from build123d import *

# Parameters (mm, degrees)
SKETCH_1_R          = 2.1
EXTRUDE_1_DEPTH     = 3
FILLET_1_R          = 3
SKETCH_2_W          = 9
SKETCH_2_H          = 5
CUT_EXTRUDE_1_DEPTH = 3
SKETCH_3_R          = 1.5
CUT_EXTRUDE_2_DEPTH = 10
FILLET_2_R          = 1.5


with BuildPart() as part:
    # 草图1 → 凸台-拉伸1 (new body)
    with BuildSketch(Plane(origin=(0, 0, 0), x_dir=(1, 0, 0), z_dir=(0, 1, 0))):
        Polygon((33, 10), (-33, 10), (-33, -10), (-10, -60), (10, -60), (33, -10), align=None)
        with Locations(Location((0, 0, 0), (0, 0, 270))):
            Circle(SKETCH_1_R, mode=Mode.SUBTRACT)
        with Locations(Location((25, 0, 0), (0, 0, 270))):
            Circle(SKETCH_1_R, mode=Mode.SUBTRACT)
        with Locations(Location((-25, 0, 0), (0, 0, 270))):
            Circle(SKETCH_1_R, mode=Mode.SUBTRACT)
        with Locations(Location((0, -25, 0), (0, 0, 270))):
            Circle(SKETCH_1_R, mode=Mode.SUBTRACT)
        with Locations(Location((0, -50, 0), (0, 0, 270))):
            Circle(SKETCH_1_R, mode=Mode.SUBTRACT)
    extrude(amount=EXTRUDE_1_DEPTH)

    # 圆角1
    fillet_1_edges = [part.edges().sort_by_distance(p)[0] for p in [
        (10, 1.5, 60),
        (-10, 1.5, 60),
        (-33, 1.5, 10),
        (-33, 1.5, -10),
        (33, 1.5, -10),
        (33, 1.5, 10),
    ]]
    fillet(fillet_1_edges, radius=FILLET_1_R)

    # 草图2 → 切除-拉伸1 (cut)
    with BuildSketch(Plane(origin=(0, 3, 0), x_dir=(1, 0, 0), z_dir=(0, 1, 0))):
        with Locations((0, -57.5)):
            Rectangle(SKETCH_2_W, SKETCH_2_H)
    extrude(amount=-CUT_EXTRUDE_1_DEPTH, mode=Mode.SUBTRACT)

    # 草图3 → 切除-拉伸2 (cut)
    with BuildSketch(Plane(origin=(0, 3, 0), x_dir=(1, 0, 0), z_dir=(0, 1, 0))):
        with Locations((-4.5, -55)):
            Circle(SKETCH_3_R)
        with Locations((4.5, -55)):
            Circle(SKETCH_3_R)
    extrude(amount=-CUT_EXTRUDE_2_DEPTH, mode=Mode.SUBTRACT)

    # 圆角2
    fillet_2_edges = [part.edges().sort_by_distance(p)[0] for p in [
        (-4.5, 1.5, 56.5),
        (3, 1.5, 55),
        (-4.5, 1.5, 60),
        (4.5, 1.5, 60),
        (4.5, 1.5, 56.5),
        (-3, 1.5, 55),
    ]]
    fillet(fillet_2_edges, radius=FILLET_2_R)


solid = part.part
Geometry check sheet. Reference: the model listing, model coordinates, mm. A direction names the side the tool comes from. Give positions to 0.01 mm unless a question says otherwise; leave off trailing zeros. Write each loop counter-clockwise with the first axis right and the second up, starting at its lowest first coordinate (ties: lowest second). Pieces come first, ordered by that corner, then holes. Notation, with made-up numbers: M -11,43 L 9,43 A6 ccw 9,50 Z; hole C -39,36.5 d11. An arc over 180 degrees is marked long. Answer as CSV lines item,"result". Start each with the question number.
Q1. Material ranges on L1, parallel to X at y = 1.6, z = 0; L2, parallel to Z at x = -1, y = 1.6; L3, parallel to X at y = 2.65, z = 57.5, recorded low to high.
Q2. Section check A-A, the plane z = 25. Record the cut outline in (x, y).
Q3. Section check B-B, the plane z = 0. Record the cut outline in (x, y).
Q4. Tool access check on faces 1 (the face through (-23.23, 1.48, 1.13)), 2 (the face through (-4.93, 1.48, 59.55)). Record the directions out of +Z, -Z, +X, -X, +Y, -Y that give a thin tool (end or side, any length) a straight path to the whole face; none if there is none.
Q5. Go/stop test with flat-tipped pins: pin 1 (4 mm diameter, centred on x = 0, z = 0, fed in from +Y); pin 2 (0.7 mm diameter, centred on y = 1, z = 58, fed in from -X); pin 3 (1 mm diameter, centred on y = 1.5, z = 58, fed in from +X). Record where each tip stops, or that it passes through.
Q6. Section check C-C, the plane x = 0. Record the cut outline in (y, z), then the cut area to 3 significant figures.
Q7. Release check for a two-part mould opening along X. For faces 3 (the face through (4.95, 1.48, 59.57)), 4 (the face through (0, 3, 17)), 5 (the face through (-32.1, 1.52, -9.14)), 6 (the face through (33, 1, 1)) record: pulls with the +X half, pulls with the -X half, needs draft (parallel to the pull), parting line crosses it, or undercut.
Q8. Section check D-D, the plane y = 2.15. Give the number of separate pieces and of enclosed holes in the cut face, then the cut area to 3 significant figures.
Geometry says:
1,L1,"-33 to -27.1, -22.9 to -2.1, 2.1 to 22.9, 27.1 to 33"
1,L2,"-10 to -1.85, 1.85 to 23.15, 26.85 to 48.15, 51.85 to 55"
1,L3,"-11.15 to -4.5, 4.5 to 11.15"
2,outline,"M -26.1,0 L -2.1,0 L -2.1,3 L -26.1,3 Z; M 2.1,0 L 26.1,0 L 26.1,3 L 2.1,3 Z"
3,outline,"M -33,0 L -27.1,0 L -27.1,3 L -33,3 Z; M -22.9,0 L -2.1,0 L -2.1,3 L -22.9,3 Z; M 2.1,0 L 22.9,0 L 22.9,3 L 2.1,3 Z; M 27.1,0 L 33,0 L 33,3 L 27.1,3 Z"
4,face 1,"+Y, -Y"
4,face 2,"+Z, +Y, -Y"
5,pin 1,"through"
5,pin 2,"x = -11.08"
5,pin 3,"x = 11.15"
6,outline,"M 0,-10 L 3,-10 L 3,-2.1 L 0,-2.1 Z; M 0,2.1 L 3,2.1 L 3,22.9 L 0,22.9 Z; M 0,27.1 L 3,27.1 L 3,47.9 L 0,47.9 Z; M 0,52.1 L 3,52.1 L 3,55 L 0,55 Z"
6,area,"157 mm^2"
7,face 3,"undercut"
7,face 4,"needs draft"
7,face 5,"pulls with the -X half"
7,face 6,"pulls with the +X half"
8,separate pieces,"1"
8,enclosed holes,"5"
8,area,"3,340 mm^2"
